Can you work these out from the drawing? Everything is in mm from the part's minimum corner. A direction names the side the tool comes from. Give positions to 0.01 mm unless a question says otherwise; leave off trailing zeros. Order: outer loops, then holes, each group sorted by start corner. A loop starts at its lowest first (then second) coordinate and runs counter-clockwise, first axis right, second up. Notation, with made-up numbers: (1.25, 5.25) -> (54.25, 5.25) arc R32 cw to (54.25, 35.25) -> close; hole circle Ø11 at (-27.75, 44). An arc over 180 degrees is marked (long way). One line per item, written item: value.
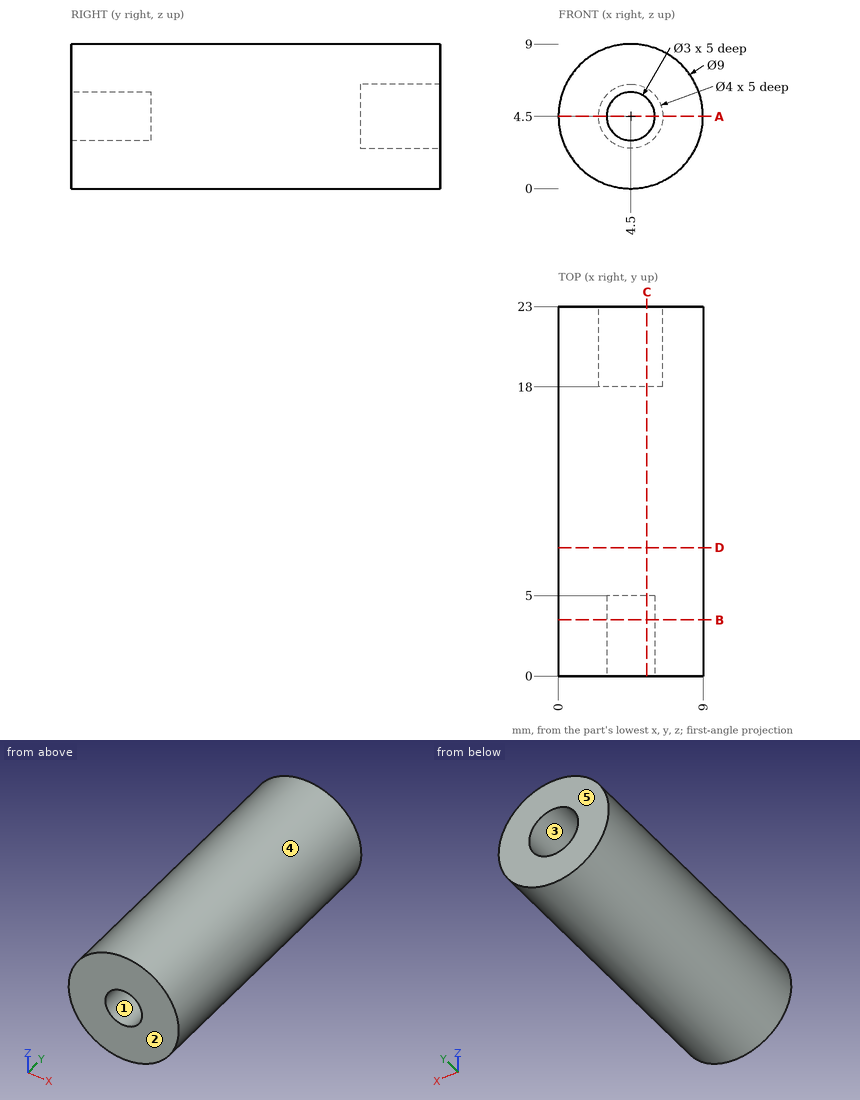
1) For P1, Ø0.9, axis at x = 5, z = 4.5, coming from the -Y side; P2, Ø3, axis at y = 16.5, z = 1.5, coming from the -X side; P3, Ø1.5, axis at x = 1, y = 16, coming from the -Z side, each with a flat end and sliding along its axis, tell me the tip position at first contact or that it passes through.
Answer below:
P1: stops at y = 5
P2: stops at x = 0.26
P3: stops at z = 0.94
2) We'd pull the mould along X, two halves only. Please class the marked faces 3, 4 and 5: +X half, -X half, draft (parallel to the pull), parting line (faces both ways), or undercut.
Answer below:
face 3: undercut
face 4: parting line
face 5: draft
3) For the marked faces 1 and 2, which set-ups out of +Z, -Z, +X, -X, +Y, -Y let a thin tool reach every point of the face, with its end or its side?
Answer below:
face 1: -Y
face 2: +Z, -Z, +X, -X, -Y
4) Suppose I cut it at D-D, the plane y = 8. Write out the boundary of the cut face in (x, z), then the cut area to 3 significant figures.
Answer below:
outline: circle Ø9 at (4.5, 4.5)
area: 63.6 mm2
5) Suppose I cut it at C-C, the plane x = 5.5. Write out the boundary of the cut face in (y, z), then the cut area to 3 significant figures.
Answer below:
outline: (0, 0.11) -> (23, 0.11) -> (23, 2.77) -> (18, 2.77) -> (18, 6.23) -> (23, 6.23) -> (23, 8.89) -> (0, 8.89) -> (0, 5.62) -> (5, 5.62) -> (5, 3.38) -> (0, 3.38) -> close
area: 173 mm2
6) Suppose I cut it at B-B, the plane y = 3.5. Write out the boundary of the cut face in (x, z).
Answer below:
outline: circle Ø9 at (4.5, 4.5); hole circle Ø3 at (4.5, 4.5)
7) If I drill on line 1 along X through (y, z) = (3.8, 4.5); line 2 along X through (y, z) = (21.85, 4.5); line 3 along Y through (x, z) = (5.25, 6), over which ranges is the centre line in solid material (lowest first)?
Answer below:
line 1: x = 0 to 3, 6 to 9
line 2: x = 0 to 2.5, 6.5 to 9
line 3: y = 0 to 18
8) Suppose I cut it at A-A, the plane z = 4.5. Write out the boundary of the cut face in (x, y).
Answer below:
outline: (0, 0) -> (3, 0) -> (3, 5) -> (6, 5) -> (6, 0) -> (9, 0) -> (9, 23) -> (6.5, 23) -> (6.5, 18) -> (2.5, 18) -> (2.5, 23) -> (0, 23) -> close
